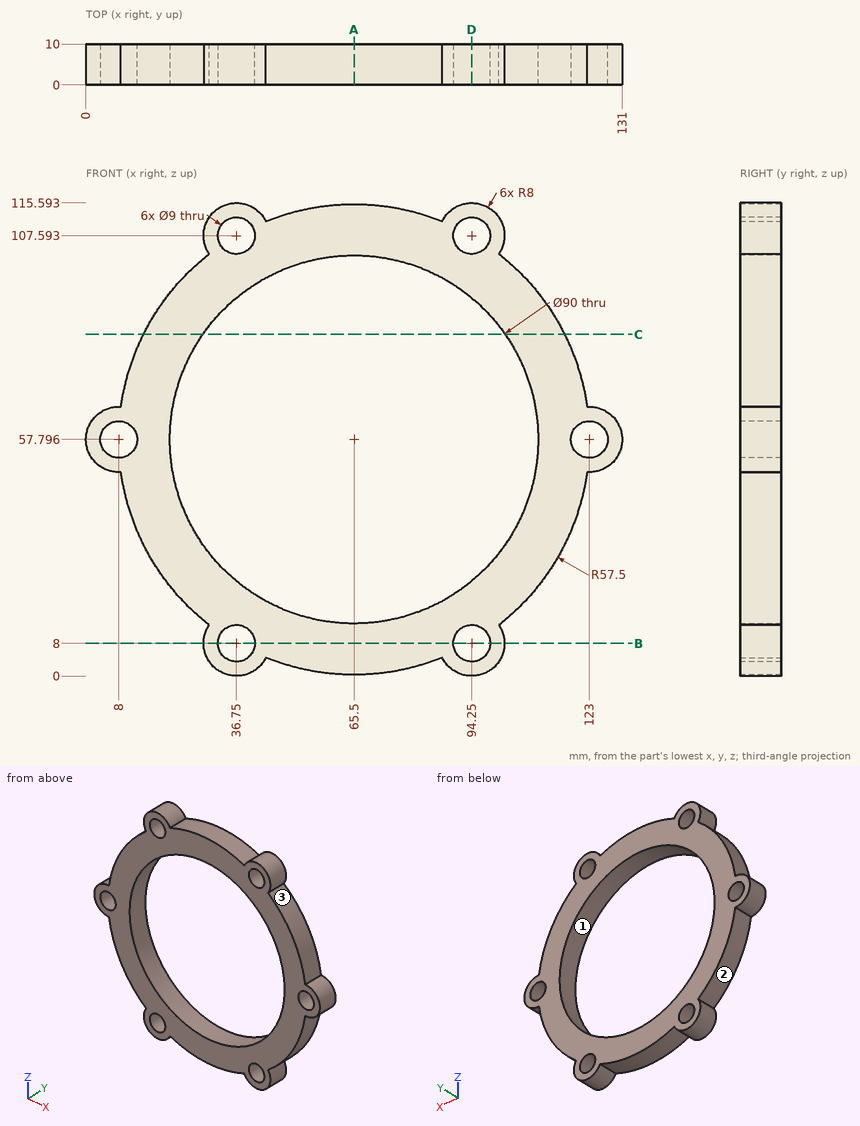
Part print with two shaded views. Sizes in mm from the minimum x, y, z corner. Coordinates: 2 decimals unless noted, no trailing zeros. Write each loop counter-clockwise with the first axis right and the second up, starting at its lowest first coordinate (ties: lowest second). Pieces come first, ordered by that corner, then holes. Notation, with made-up numbers: (-36, 87.25) - (-6, 87.25) arc R24 cw to (-6, 116.25) - close; hole circle Ø4 at (77, 74). An arc over 180 degrees is marked (long way). Use a Markdown table: item, result. Add a question column.
Item 1: Two-plate mould, pull along X, no slides. Class the marked faces 1, 2 and 3: pulls with the +X half, pulls with the -X half, needs draft (parallel to the pull), parting line crosses it, or undercut.
Item 2: Band-saw the part on C-C, the plane z = 83.5. Write the cut outline in (x, y) (1 decimal), and give its area (3 significant figures).
Item 3: Band-saw the part on D-D, the plane x = 94.25. Write the cut outline in (y, z) (1 decimal).
Item 4: Band-saw the part on A-A, the plane x = 65.5. Write the cut outline in (y, z), and give its area (3 significant figures).
Item 5: Drop flat-ended pins along their axis: pin 1 (5 mm diameter, centred on x = 100, y = 7, fed in from -Z); pin 2 (4 mm diameter, centred on x = 97.5, y = 8.5, fed in from -Z); pin 3 (4 mm diameter, centred on x = 103, y = 4.5, fed in from -Z) (1 decimal). Give the stop position or say it passes through.
Item 6: Band-saw the part on B-B, the plane z = 8. Write the cut outline in (x, y), and give its area (3 significant figures).
Item 7: Drill centre lines: line 1 along X through (y, z) = (3.5, 8); line 2 along Z through (x, y) = (8, 4.5); line 3 along X through (y, z) = (5.25, 10.5). Where is each one in solid material? Low to high.
A:
| question | item | result |
|---|---|---|
| 1 | face 1 | undercut |
| 1 | face 2 | pulls with the -X half |
| 1 | face 3 | pulls with the +X half |
| 2 | outline | (14.1, 0) - (28.6, 0) - (28.6, 10) - (14.1, 10) - close; (102.4, 0) - (116.9, 0) - (116.9, 10) - (102.4, 10) - close |
| 2 | area | 290 mm² |
| 3 | outline | (0, 0) - (10, 0) - (10, 3.5) - (0, 3.5) - close; (0, 12.5) - (10, 12.5) - (10, 23.2) - (0, 23.2) - close; (0, 92.4) - (10, 92.4) - (10, 103.1) - (0, 103.1) - close; (0, 112.1) - (10, 112.1) - (10, 115.6) - (0, 115.6) - close |
| 4 | outline | (0, 0.3) - (10, 0.3) - (10, 12.8) - (0, 12.8) - close; (0, 102.8) - (10, 102.8) - (10, 115.3) - (0, 115.3) - close |
| 4 | area | 250 mm² |
| 5 | pin 1 | stops at z = 0.69 |
| 5 | pin 2 | stops at z = 0.1 |
| 5 | pin 3 | stops at z = 3.7 |
| 6 | outline | (28.75, 0) - (32.25, 0) - (32.25, 10) - (28.75, 10) - close; (41.25, 0) - (89.75, 0) - (89.75, 10) - (41.25, 10) - close; (98.75, 0) - (102.25, 0) - (102.25, 10) - (98.75, 10) - close |
| 6 | area | 555 mm² |
| 7 | line 1 | x = 28.75 to 32.25, 41.25 to 89.75, 98.75 to 102.25 |
| 7 | line 2 | z = 49.8 to 53.3, 62.3 to 65.8 |
| 7 | line 3 | x = 29.15 to 33.01, 40.49 to 90.51, 97.99 to 101.85 |
